Verification items for the finished model (mm, model axes). Coordinates: 2 decimals unless noted, no trailing zeros. Order: outer loops, then holes, each group sorted by start corner. A loop starts at its lowest first (then second) coordinate and runs counter-clockwise, first axis right, second up. Notation, with made-up numbers: (7, 5.5) -> (56, 5.5) arc R24 ccw to (56, 20.5) -> close; hole circle Ø7 at (27.25, 64). An arc over 180 degrees is marked (long way). Answer as CSV lines item,"result".
```python
from build123d import *

# Parameters (mm, degrees)
SKETCH_R   = 0.6
SKETCH_W   = 1
SKETCH_H   = 37.72
SKETCH_H_2 = 21.76
SKETCH_W_2 = 19.7
SKETCH_H_3 = 1.2
SKETCH_W_3 = 12.5
SKETCH_H_4 = 1
SKETCH_W_4 = 20
PAD_DEPTH  = 1.6


with BuildPart() as part:
    # Sketch → Pad (new body)
    with BuildSketch(Plane.XY):
        with BuildLine():
            Line((-30.13, 22.36), (30.13, 22.36))
            ThreePointArc((33.13, 19.36), (32.25132, 21.48132), (30.13, 22.36))
            Line((33.13, 19.36), (33.13, -19.36))
            ThreePointArc((30.13, -22.36), (32.25132, -21.48132), (33.13, -19.36))
            Line((28.13, -22.36), (30.13, -22.36))
            Line((28.13, -22.36), (28.13, -27.36))
            Line((28.13, -27.36), (30.13, -27.36))
            ThreePointArc((33.13, -30.36), (32.25132, -28.23868), (30.13, -27.36))
            Line((33.13, -30.36), (33.13, -47.26))
            ThreePointArc((30.13, -50.26), (32.25132, -49.38132), (33.13, -47.26))
            Line((30.13, -50.26), (9.43, -50.26))
            ThreePointArc((6.43, -47.26), (7.30868, -49.38132), (9.43, -50.26))
            Line((6.43, -47.26), (6.43, -30.36))
            ThreePointArc((9.43, -27.36), (7.30868, -28.23868), (6.43, -30.36))
            Line((9.43, -27.36), (20.13, -27.36))
            Line((20.13, -27.36), (20.13, -22.36))
            Line((20.13, -22.36), (-20.13, -22.36))
            Line((-20.13, -22.36), (-20.13, -27.36))
            Line((-20.13, -27.36), (-0.91, -27.36))
            ThreePointArc((2.09, -30.36), (1.21132, -28.23868), (-0.91, -27.36))
            Line((2.09, -30.36), (2.09, -52.52))
            ThreePointArc((-0.91, -55.52), (1.21132, -54.64132), (2.09, -52.52))
            Line((-30.13, -55.52), (-0.91, -55.52))
            ThreePointArc((-33.13, -52.519977), (-32.251329, -54.641312), (-30.13, -55.52))
            Line((-33.13, -52.519977), (-33.13, -50.519977))
            Line((-33.13, -50.519977), (-34.83, -50.519977))
            Line((-34.83, -52.519977), (-34.83, -50.519977))
            ThreePointArc((-37.83, -55.52), (-35.708671, -54.641312), (-34.83, -52.519977))
            Line((-37.83, -55.52), (-63.9, -55.52))
            ThreePointArc((-66.9, -52.52), (-66.02132, -54.64132), (-63.9, -55.52))
            Line((-66.9, -52.52), (-66.9, -15.09))
            ThreePointArc((-63.9, -12.09), (-66.02132, -12.96868), (-66.9, -15.09))
            Line((-63.9, -12.09), (-37.83, -12.09))
            ThreePointArc((-34.83, -15.09), (-35.70868, -12.96868), (-37.83, -12.09))
            Line((-34.83, -15.09), (-34.83, -45.519977))
            Line((-33.13, -45.519977), (-34.83, -45.519977))
            Line((-33.13, -30.36), (-33.13, -45.519977))
            ThreePointArc((-30.13, -27.36), (-32.25132, -28.23868), (-33.13, -30.36))
            Line((-28.13, -27.36), (-30.13, -27.36))
            Line((-28.13, -22.36), (-28.13, -27.36))
            Line((-30.13, -22.36), (-28.13, -22.36))
            ThreePointArc((-33.13, -19.36), (-32.25132, -21.48132), (-30.13, -22.36))
            Line((-33.13, -17.86), (-33.13, -19.36))
            Line((-33.13, 9.36), (-33.13, -17.86))
            Line((-33.13, 9.36), (-38.13, 9.36))
            Line((-38.13, -6.59), (-38.13, 9.36))
            ThreePointArc((-41.13, -9.59), (-39.00868, -8.71132), (-38.13, -6.59))
            Line((-41.13, -9.59), (-54.63, -9.59))
            ThreePointArc((-57.63, -6.59), (-56.75132, -8.71132), (-54.63, -9.59))
            Line((-57.63, -6.59), (-57.63, 19.36))
            ThreePointArc((-54.63, 22.36), (-56.75132, 21.48132), (-57.63, 19.36))
            Line((-54.63, 22.36), (-41.13, 22.36))
            ThreePointArc((-38.13, 19.36), (-39.00868, 21.48132), (-41.13, 22.36))
            Line((-38.13, 19.36), (-38.13, 17.36))
            Line((-38.13, 17.36), (-33.13, 17.36))
            Line((-33.13, 19.405686), (-33.13, 17.36))
            ThreePointArc((-30.13, 22.36), (-32.23523, 21.497432), (-33.13, 19.405686))
        make_face()
        with Locations((-31.33, 20.36)):
            Circle(SKETCH_R, mode=Mode.SUBTRACT)
        with Locations((-31.33, -20.36)):
            Circle(SKETCH_R, mode=Mode.SUBTRACT)
        with Locations((31.33, 20.36)):
            Circle(SKETCH_R, mode=Mode.SUBTRACT)
        with Locations((31.33, -20.36)):
            Circle(SKETCH_R, mode=Mode.SUBTRACT)
        with Locations((-31.33, -29.36)):
            Circle(SKETCH_R, mode=Mode.SUBTRACT)
        with Locations((-31.33, -53.52)):
            Circle(SKETCH_R, mode=Mode.SUBTRACT)
        with Locations((0.29, -29.36)):
            Circle(SKETCH_R, mode=Mode.SUBTRACT)
        with Locations((0.29, -53.52)):
            Circle(SKETCH_R, mode=Mode.SUBTRACT)
        with Locations((8.43, -48.46)):
            Circle(SKETCH_R, mode=Mode.SUBTRACT)
        with Locations((31.13, -29.16)):
            Circle(SKETCH_R, mode=Mode.SUBTRACT)
        with Locations((31.13, -48.46)):
            Circle(SKETCH_R, mode=Mode.SUBTRACT)
        with Locations((8.43, -29.16)):
            Circle(SKETCH_R, mode=Mode.SUBTRACT)
        with Locations((-55.83, 20.36)):
            Circle(SKETCH_R, mode=Mode.SUBTRACT)
        with Locations((-39.93, -7.59)):
            Circle(SKETCH_R, mode=Mode.SUBTRACT)
        with Locations((-55.83, -7.59)):
            Circle(SKETCH_R, mode=Mode.SUBTRACT)
        with Locations((-39.93, 20.36)):
            Circle(SKETCH_R, mode=Mode.SUBTRACT)
        with Locations((-64.9, -13.89)):
            Circle(SKETCH_R, mode=Mode.SUBTRACT)
        with Locations((-36.83, -13.89)):
            Circle(SKETCH_R, mode=Mode.SUBTRACT)
        with Locations((-36.83, -53.72)):
            Circle(SKETCH_R, mode=Mode.SUBTRACT)
        with Locations((-64.9, -53.72)):
            Circle(SKETCH_R, mode=Mode.SUBTRACT)
        with Locations((30.13, 0)):
            Rectangle(SKETCH_W, SKETCH_H, mode=Mode.SUBTRACT)
        with Locations((-0.41, -41.44)):
            Rectangle(SKETCH_W, SKETCH_H_2, mode=Mode.SUBTRACT)
        with Locations((19.78, -47.86)):
            Rectangle(SKETCH_W_2, SKETCH_H_3, mode=Mode.SUBTRACT)
        with Locations((-47.88, -7.09)):
            Rectangle(SKETCH_W_3, SKETCH_H_4, mode=Mode.SUBTRACT)
        with Locations((-50.865, -53.02)):
            Rectangle(SKETCH_W_4, SKETCH_H_4, mode=Mode.SUBTRACT)
    extrude(amount=PAD_DEPTH)


solid = part.part
```
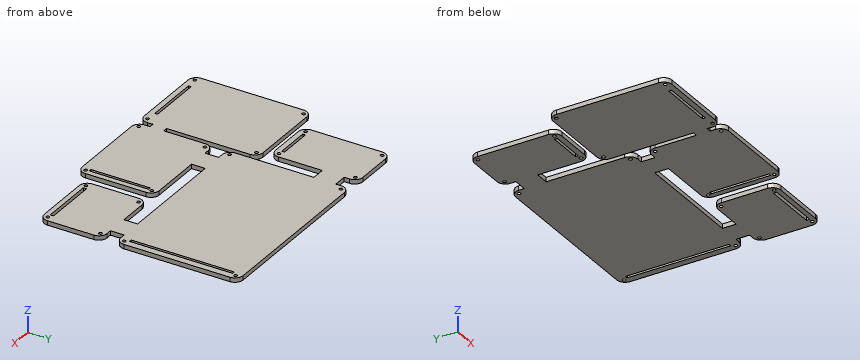
Item 1: Section check C-C, the plane x = 15. Record the boundary of the cut face in (y, z), plus the area to 3 significant figures.
Answer list:
outline,"(-50.26, 0) -> (-48.46, 0) -> (-48.46, 1.6) -> (-50.26, 1.6) -> close; (-47.26, 0) -> (-27.36, 0) -> (-27.36, 1.6) -> (-47.26, 1.6) -> close; (-22.36, 0) -> (22.36, 0) -> (22.36, 1.6) -> (-22.36, 1.6) -> close"
area,"106 mm2"
Item 2: Section check B-B, the plane y = -32. Record the boundary of the cut face in (x, z).
Answer list:
outline,"(-66.9, 0) -> (-34.83, 0) -> (-34.83, 1.6) -> (-66.9, 1.6) -> close; (-33.13, 0) -> (-0.91, 0) -> (-0.91, 1.6) -> (-33.13, 1.6) -> close; (0.09, 0) -> (2.09, 0) -> (2.09, 1.6) -> (0.09, 1.6) -> close; (6.43, 0) -> (33.13, 0) -> (33.13, 1.6) -> (6.43, 1.6) -> close"
Item 3: Section check A-A, the plane x = -44.5. Record the boundary of the cut face in (y, z).
Answer list:
outline,"(-55.52, 0) -> (-53.52, 0) -> (-53.52, 1.6) -> (-55.52, 1.6) -> close; (-52.52, 0) -> (-12.09, 0) -> (-12.09, 1.6) -> (-52.52, 1.6) -> close; (-9.59, 0) -> (-7.59, 0) -> (-7.59, 1.6) -> (-9.59, 1.6) -> close; (-6.59, 0) -> (22.36, 0) -> (22.36, 1.6) -> (-6.59, 1.6) -> close"
Item 4: Section check D-D, the plane z = 0.75. Count the separate pieces of the cut face and the enclosed holes in it, plus the area to 3 significant figures.
Answer list:
separate pieces,"1"
enclosed holes,"25"
area,"6,530 mm2"
Item 5: Depth check by flat-ended pin: pin 1 Ø0.5 at (x, z) = (-0.5, 0.5) entering from -Y. Enter the tip coordinate at first touch or a pass-through.
Answer list:
pin 1,"y = -55.52"
Item 6: Thickness scan on line 1 (X direction, y = -4, z = 1.45); line 2 (X direction, y = -27, z = 0.25); line 3 (Y direction, x = -55, z = 1.5). Record the ranges inside material, lowest first.
Answer list:
line 1,"-57.63 to -38.13, -33.13 to 29.63, 30.63 to 33.13"
line 2,"-66.9 to -34.83, -28.13 to -20.13, 20.13 to 28.13"
line 3,"-55.52 to -53.52, -52.52 to -12.09, -9.57 to 22.34"
